Print and shaded views of the part. All mm, measured from the part's lowest x, y and z. A direction names the side the tool comes from. Round coordinates to 2 decimals unless told otherwise and drop trailing zeros. Write each loop counter-clockwise with the first axis right and the second up, starting at its lowest first coordinate (ties: lowest second). Pieces come first, ordered by that corner, then holes. Notation, with made-up numbers: M 49,31.25 L 84,31.25 A21 cw 84,62.25 Z; hole C 56.25,-1 d5. An arc over 180 degrees is marked long. Write item = value, one per line.
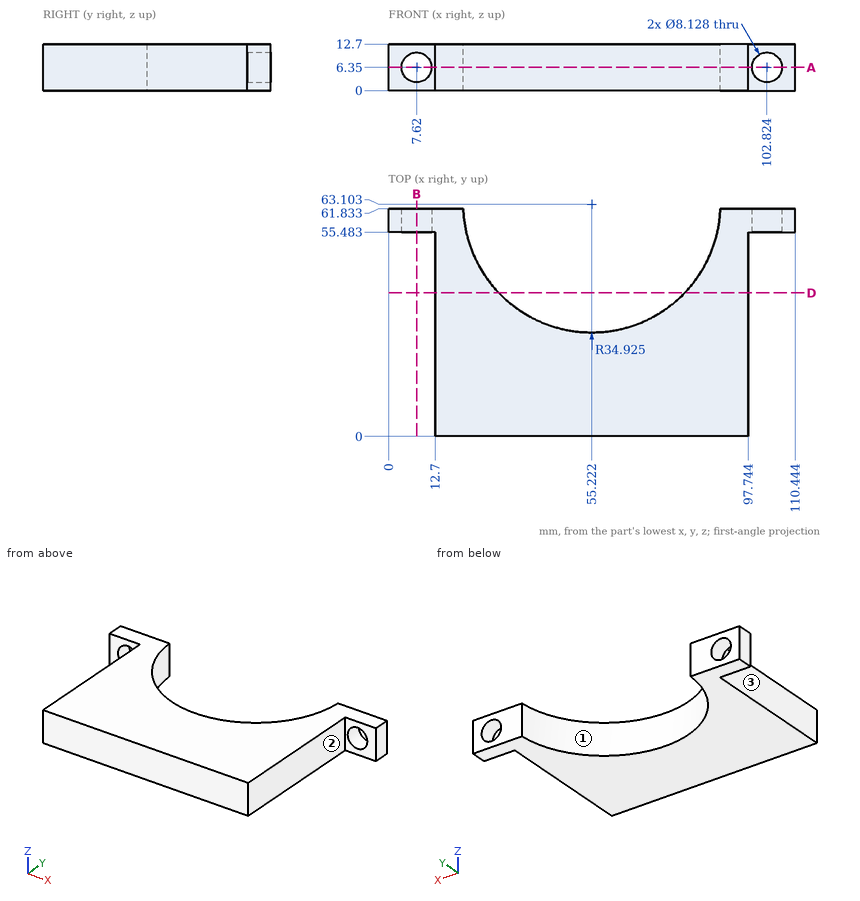
1. Band-saw the part on D-D (y = 39). List the corners of the cut face in (x, z), plus the area to 3 significant figures.
Responses:
outline = M 12.7,0 L 29.95,0 L 29.95,12.7 L 12.7,12.7 Z; M 80.5,0 L 97.74,0 L 97.74,12.7 L 80.5,12.7 Z
area = 438 mm²
2. Probe probe 1 along X at (y, z) = (59.5, 6.35); probe 2 along X at (y, z) = (59, 6.35) (1 decimal); probe 3 along X at (y, z) = (25.5, 6.25). List the from-to ranges inside material, lowest first.
Responses:
probe_1 = 0 to 3.56, 11.68 to 20.48, 89.96 to 98.76, 106.89 to 110.44
probe_2 = 0 to 3.6, 11.7 to 20.5, 89.9 to 98.8, 106.9 to 110.4
probe_3 = 12.7 to 97.74
3. Band-saw the part on B-B (x = 7.62). List the corners of the cut face in (y, z).
Responses:
outline = M 55.48,0 L 61.83,0 L 61.83,2.29 L 55.48,2.29 Z; M 55.48,10.41 L 61.83,10.41 L 61.83,12.7 L 55.48,12.7 Z
4. Tool access for the marked faces 1, 2 and 3: list every direction of +Z, -Z, +X, -X, +Y, -Y with a clear straight run to the whole face (end or side of a thin tool).
Responses:
face_1 = +Z, -Z, +Y
face_2 = +Z, -Z, +X, -Y
face_3 = +Z, -Z, -X, -Y
5. Flat gauge pins, fed straight in: pin 1 (4 mm diameter, centred on y = 17, z = 7.5, fed in from -X); pin 2 (4 mm diameter, centred on y = 26, z = 4.5, fed in from +X). Where does each tip first touch, or does it go through?
Responses:
pin_1 = 12.7
pin_2 = 97.74
6. Band-saw the part on A-A (z = 6.35). Count the separate pieces of the cut face and the enclosed holes in it, plus the area to 3 significant figures.
Responses:
separate_pieces = 3
enclosed_holes = 0
area = 3,490 mm²
